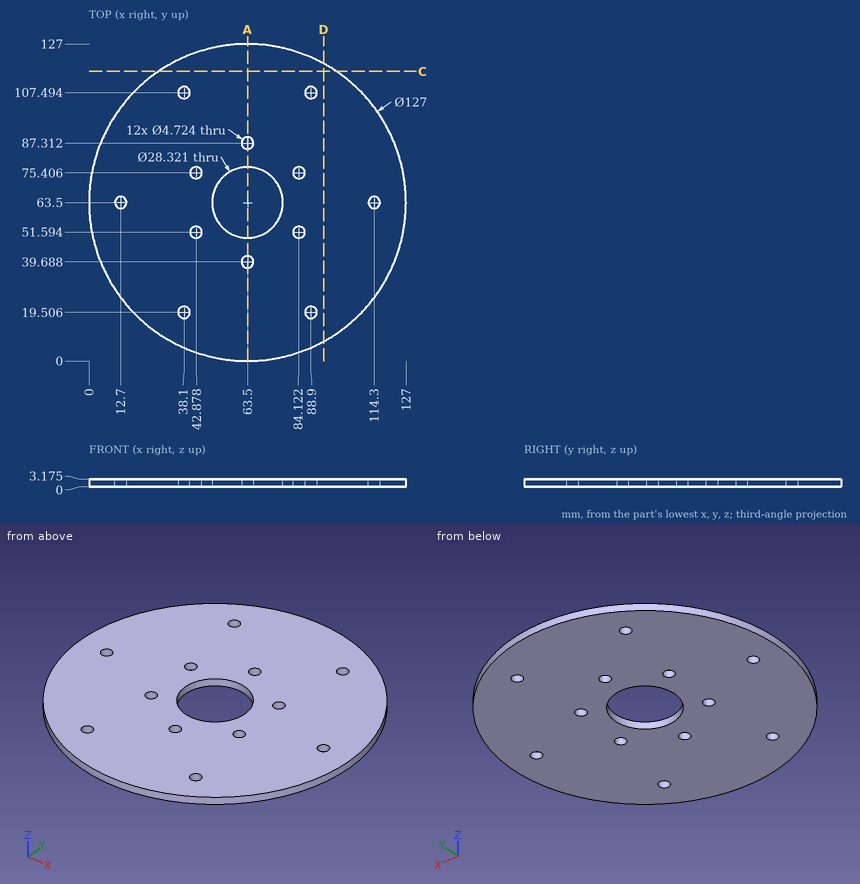
Study the drawing (mm; zero at the part's minimum x, y, z) and answer. Give positions to 0.01 mm unless a question says otherwise; leave off trailing zeros. Order: outer loops, then holes, each group sorted by start corner. A loop starts at its lowest first (then second) coordinate and runs counter-clockwise, first axis right, second up. Notation, with made-up numbers: M -28.75,89.5 L -3.75,89.5 A19 ccw -3.75,115.5 Z; hole C -31,37.25 d1. An arc over 180 degrees is marked long. Put each result on its own line as item: value. Start each with the question number.
Item 1: The part is cut by section A-A, the plane x = 63.5. State how many separate pieces and enclosed holes the cut face has.
Item 2: The part is cut by section C-C, the plane y = 116. Determine the outline of the cut face in (x, z) (1 decimal).
Item 3: The part is cut by section D-D, the plane x = 94. Determine the outline of the cut face in (y, z) (1 decimal).
Item 4: Find the intervals of material crossed by line 1 along Y through (x, z) = (87, 2.6) (1 decimal); line 2 along Y through (x, z) = (88.9, 1.35) (1 decimal); line 3 along X through (y, z) = (39, 0.95) (1 decimal), in increasing order.
Item 5: Flat-ended cylindrical pins translate along their axes: P1, Ø4, axis at x = 38.1, y = 19.51, coming from the -Z side; P2, Ø1, axis at x = 94, z = 1, coming from the +Y side; P3, Ø1.5, axis at x = 17.5, z = 1.5, coming from the -Y side; P4, Ø1, axis at x = 23, z = 0.5, coming from the +Y side. Find the tip coordinate at first contact, or state that the pin passes through.
Answer key:
1. separate pieces: 4
1. enclosed holes: 0
2. outline: M 27.8,0 L 99.2,0 L 99.2,3.2 L 27.8,3.2 Z
3. outline: M 7.8,0 L 119.2,0 L 119.2,3.2 L 7.8,3.2 Z
4. line 1: y = 4.5 to 18.1, 20.9 to 106.1, 108.9 to 122.5
4. line 2: y = 5.3 to 17.1, 21.9 to 105.1, 109.9 to 121.7
4. line 3: x = 4.9 to 61.2, 65.8 to 122.1
5. P1: passes through
5. P2: stops at y = 119.47
5. P3: stops at y = 18.95
5. P4: stops at y = 112.82
